CAD build for the part. Positions are in the model's coordinates, mm. Round coordinates to 2 decimals unless told otherwise and drop trailing zeros. Order: outer loops, then holes, each group sorted by start corner. A loop starts at its lowest first (then second) coordinate and runs counter-clockwise, first axis right, second up.
```python
from build123d import *


with BuildPart() as f1:
    # F0 (on Front) → F1 (revolve)
    with BuildSketch(Plane.XZ):
        with BuildLine():
            Line((4, 3.25), (4, 0))
            Line((4, 0), (5, 0))
            ThreePointArc((5, 0), (5.263932, 1.118034), (6, 2))
            Line((6, 2), (6, 3.25))
            ThreePointArc((6, 3.25), (5.926777, 3.426777), (5.75, 3.5))
            Line((5.75, 3.5), (4.25, 3.5))
            ThreePointArc((4.25, 3.5), (4.073223, 3.426777), (4, 3.25))
        make_face()
        with BuildLine():
            Line((5, 0), (4, 0))
            Line((4, 0), (4, -3.25))
            ThreePointArc((4, -3.25), (4.073223, -3.426777), (4.25, -3.5))
            Line((4.25, -3.5), (5.75, -3.5))
            ThreePointArc((5.75, -3.5), (5.926777, -3.426777), (6, -3.25))
            Line((6, -3.25), (6, -2))
            ThreePointArc((6, -2), (5.263932, -1.118034), (5, 0))
        make_face()
    revolve(axis=Axis((0, 0, 0.334755), (0, 0, -1)))


solid = f1.part
```
1. Cut at B-B, the plane z = -0.5. Write the cut outline in (x, y), and give its area (3 significant figures).
2. Cut at A-A, the plane z = 1. Write the cut outline in (x, y), and give its area (3 significant figures).
3. Drill centre lines: line 1 (X direction, y = 3.25, z = -0.5); line 2 (X direction, y = 0, z = 1.75); line 3 (Y direction, x = 0, z = -1.5). Where is each one in solid material? Low to high.
4. Pin check, flat tips, straight feed: P1, Ø1.5, axis at y = -2, z = 2, coming from the -X side; P2, Ø1.5, axis at x = -2, z = -1.5, coming from the -Y side; P3, Ø4, axis at y = 3, z = -0.5, coming from the -X side. Stop position of each tip, or through.
5. Mould opens along X. For faces 1 (the face through (-0.867, 3.905, -0.046)), 2 (the face through (-6, 0, 3)), 3 (the face through (-2, 4, 3.5)) say: released by +X, released by -X, zero draft, split by the parting line, or undercut.
Outcome:
1. outline: circle Ø10.1 at (0, 0); hole circle Ø8 at (0, 0)
1. area: 29.9 mm2
2. outline: circle Ø10.42 at (0, 0); hole circle Ø8 at (0, 0)
2. area: 35.0 mm2
3. line 1: x = -3.87 to -2.33, 2.33 to 3.87
3. line 2: x = -5.71 to -4, 4 to 5.71
3. line 3: y = -5.5 to -4, 4 to 5.5
4. P1: stops at x = -5.87
4. P2: stops at y = -5.82
4. P3: stops at x = -5.76
5. face 1: undercut
5. face 2: split by the parting line
5. face 3: zero draft
